The listing builds one solid part. Answer for the finished solid, in the listing's coordinates (mm). Give positions to 0.01 mm unless a question says otherwise; leave off trailing zeros. Write each loop counter-clockwise with the first axis right and the second up, starting at its lowest first coordinate (ties: lowest second). Pieces come first, ordered by that corner, then holes. Notation, with made-up numbers: M -9,-15.5 L 7,-15.5 A27 cw 7,21.5 Z; hole C 59.5,-18 d5. An arc over 180 degrees is marked long. Return JSON: item names as keys, results as strings.
from build123d import *

# Parameters (mm, degrees)
F0_W     = 435
F0_H     = 176
F0_R     = 2.5
F0_W_2   = 53.5
F0_H_2   = 13
F0_R_2   = 3.25
F0_R_3   = 4.5
F0_R_4   = 1.5
F0_W_3   = 7
F0_H_3   = 14.5
F0_R_5   = 8
F0_R_6   = 1.75
F1_DEPTH = 2


with BuildPart() as f1:
    # F0 (on Top) → F1 (new body)
    with BuildSketch(Plane.XY):
        Rectangle(F0_W, F0_H)
        with Locations((-211.722836, -80)):
            Circle(F0_R, mode=Mode.SUBTRACT)
        with Locations((-175.25, -63.5)):
            Rectangle(F0_W_2, F0_H_2, mode=Mode.SUBTRACT)
        with Locations((-115.75, -63.5)):
            Rectangle(F0_W_2, F0_H_2, mode=Mode.SUBTRACT)
        with Locations((-42.060282, -46.764122)):
            Circle(F0_R_2, mode=Mode.SUBTRACT)
        with Locations((-42.060282, -21.764122)):
            Circle(F0_R_2, mode=Mode.SUBTRACT)
        with Locations((52.5, -53)):
            Circle(F0_R_3, mode=Mode.SUBTRACT)
        with Locations((72.5, -53)):
            Circle(F0_R_3, mode=Mode.SUBTRACT)
        with Locations((92.5, -53)):
            Circle(F0_R_3, mode=Mode.SUBTRACT)
        with Locations((112.5, -53)):
            Circle(F0_R_3, mode=Mode.SUBTRACT)
        with Locations((132.5, -53)):
            Circle(F0_R_3, mode=Mode.SUBTRACT)
        with Locations((152.5, -53)):
            Circle(F0_R_3, mode=Mode.SUBTRACT)
        with Locations((172.5, -53)):
            Circle(F0_R_3, mode=Mode.SUBTRACT)
        with Locations((192.5, -53)):
            Circle(F0_R_3, mode=Mode.SUBTRACT)
        with Locations((52.5, -33)):
            Circle(F0_R_3, mode=Mode.SUBTRACT)
        with Locations((72.5, -33)):
            Circle(F0_R_3, mode=Mode.SUBTRACT)
        with Locations((92.5, -33)):
            Circle(F0_R_3, mode=Mode.SUBTRACT)
        with Locations((52.5, -13)):
            Circle(F0_R_3, mode=Mode.SUBTRACT)
        with Locations((72.5, -13)):
            Circle(F0_R_3, mode=Mode.SUBTRACT)
        with Locations((92.5, -13)):
            Circle(F0_R_3, mode=Mode.SUBTRACT)
        with Locations((112.5, -33)):
            Circle(F0_R_3, mode=Mode.SUBTRACT)
        with Locations((132.5, -33)):
            Circle(F0_R_3, mode=Mode.SUBTRACT)
        with Locations((152.5, -33)):
            Circle(F0_R_3, mode=Mode.SUBTRACT)
        with Locations((172.5, -33)):
            Circle(F0_R_3, mode=Mode.SUBTRACT)
        with Locations((192.5, -33)):
            Circle(F0_R_3, mode=Mode.SUBTRACT)
        with Locations((112.5, -13)):
            Circle(F0_R_3, mode=Mode.SUBTRACT)
        with Locations((132.5, -13)):
            Circle(F0_R_3, mode=Mode.SUBTRACT)
        with Locations((152.5, -13)):
            Circle(F0_R_3, mode=Mode.SUBTRACT)
        with Locations((172.5, -13)):
            Circle(F0_R_3, mode=Mode.SUBTRACT)
        with Locations((192.5, -13)):
            Circle(F0_R_3, mode=Mode.SUBTRACT)
        with Locations((-42.060282, 3.235878)):
            Circle(F0_R_2, mode=Mode.SUBTRACT)
        with Locations((-42.060282, 28.235878)):
            Circle(F0_R_2, mode=Mode.SUBTRACT)
        with Locations((-202, 47.721983)):
            Circle(F0_R_4, mode=Mode.SUBTRACT)
        with Locations((-202, 62.771983)):
            Rectangle(F0_W_3, F0_H_3, mode=Mode.SUBTRACT)
        with Locations((-202, 77.821983)):
            Circle(F0_R_4, mode=Mode.SUBTRACT)
        with Locations((-42.060282, 53.235878)):
            Circle(F0_R_2, mode=Mode.SUBTRACT)
        with Locations((52.5, 7)):
            Circle(F0_R_3, mode=Mode.SUBTRACT)
        with Locations((72.5, 7)):
            Circle(F0_R_3, mode=Mode.SUBTRACT)
        with Locations((92.5, 7)):
            Circle(F0_R_3, mode=Mode.SUBTRACT)
        with Locations((0, 28.235878)):
            Circle(F0_R_2, mode=Mode.SUBTRACT)
        with Locations((52.5, 27)):
            Circle(F0_R_3, mode=Mode.SUBTRACT)
        with Locations((72.5, 27)):
            Circle(F0_R_3, mode=Mode.SUBTRACT)
        with Locations((92.5, 27)):
            Circle(F0_R_3, mode=Mode.SUBTRACT)
        with Locations((112.5, 7)):
            Circle(F0_R_3, mode=Mode.SUBTRACT)
        with Locations((132.5, 7)):
            Circle(F0_R_3, mode=Mode.SUBTRACT)
        with Locations((152.5, 7)):
            Circle(F0_R_3, mode=Mode.SUBTRACT)
        with Locations((172.5, 7)):
            Circle(F0_R_3, mode=Mode.SUBTRACT)
        with Locations((192.5, 7)):
            Circle(F0_R_3, mode=Mode.SUBTRACT)
        with Locations((112.5, 27)):
            Circle(F0_R_3, mode=Mode.SUBTRACT)
        with Locations((132.5, 27)):
            Circle(F0_R_3, mode=Mode.SUBTRACT)
        with Locations((152.5, 27)):
            Circle(F0_R_3, mode=Mode.SUBTRACT)
        with Locations((172.5, 27)):
            Circle(F0_R_3, mode=Mode.SUBTRACT)
        with Locations((192.5, 27)):
            Circle(F0_R_3, mode=Mode.SUBTRACT)
        with Locations((0, 53.235878)):
            Circle(F0_R_5, mode=Mode.SUBTRACT)
        with Locations((163.5, 63)):
            Circle(F0_R_6, mode=Mode.SUBTRACT)
        with BuildLine():
            ThreePointArc((197.5, 57), (196.328427, 54.171573), (193.5, 53))
            Line((193.5, 53), (173.5, 53))
            ThreePointArc((173.5, 53), (170.671573, 54.171573), (169.5, 57))
            Line((169.5, 57), (169.5, 69))
            ThreePointArc((169.5, 69), (170.671573, 71.828427), (173.5, 73))
            Line((173.5, 73), (193.5, 73))
            ThreePointArc((193.5, 73), (196.328427, 71.828427), (197.5, 69))
            Line((197.5, 69), (197.5, 57))
        make_face(mode=Mode.SUBTRACT)
        with Locations((203.5, 63)):
            Circle(F0_R_6, mode=Mode.SUBTRACT)
    extrude(amount=-F1_DEPTH)


solid = f1.part
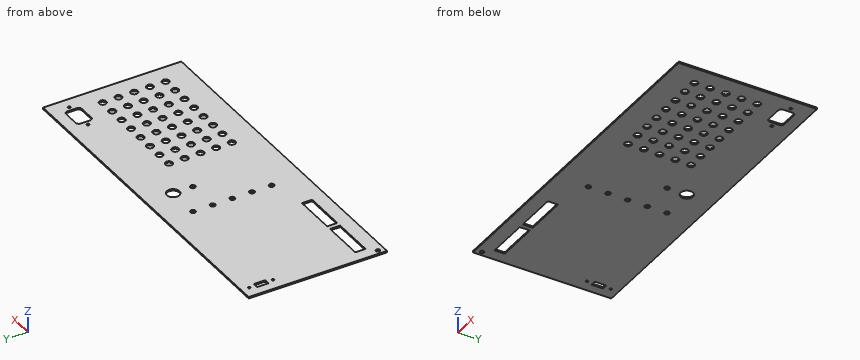
Item 1: Given pin 1 Ø1.5 at (x, y) = (-92.5, -4.5) entering from +Z; pin 2 Ø2.5 at (x, y) = (-202, 77.82) entering from -Z, each flat-ended and moving along its own axis, determine where each tip first touches the part or whether it passes through.
Geometry results:
{"pin 1": "stops at z = 0", "pin 2": "passes through"}
Item 2: A cutting plane is placed at B-B, the plane y = -13. Count the separate pieces of the cut face and the enclosed holes in it, plus the area to 3 significant figures.
Geometry results:
{"separate pieces": "9", "enclosed holes": "0", "area": "726 mm2"}
Item 3: Find the intervals of material crossed by line 1 (Y direction, x = 92.5, z = -0.9); line 2 (X direction, y = -60, z = -0.65); line 3 (Y direction, x = -192, z = -1.4), in increasing order.
Geometry results:
{"line 1": "y = -88 to -57.5, -48.5 to -37.5, -28.5 to -17.5, -8.5 to 2.5, 11.5 to 22.5, 31.5 to 88", "line 2": "x = -217.5 to -202, -148.5 to -142.5, -89 to 217.5", "line 3": "y = -88 to -70, -57 to 88"}
Item 4: A cutting plane is placed at A-A, the plane x = -105.5. Write down the section's boundary in (y, z).
Geometry results:
{"outline": "M -88,-2 L -70,-2 L -70,0 L -88,0 Z; M -57,-2 L 88,-2 L 88,0 L -57,0 Z"}
